Geometry: final body of the model. Coordinates: model frame, mm. A direction names the side the tool comes from. Give positions to 0.01 mm unless a question says otherwise; leave off trailing zeros. Write each loop counter-clockwise with the first axis right and the second up, starting at its lowest first coordinate (ties: lowest second). Pieces come first, ordered by that corner, then holes. Notation, with made-up numbers: (50, -18.75) -> (102, -18.75) arc R22 ccw to (102, 10.25) -> close; hole circle Ø1 at (3, -38.75). An arc over 180 degrees is marked (long way). Answer in a Markdown table with one row per item. Add a question column.
Item 1: Access query for faces 5 (the cylindrical face through (19.56, -1.13, -14.12)), 6 (the flat face through (-10.75, -1, -32)). Directions: +Z, -Z, +X, -X, +Y, -Y. A direction counts if a zero-diameter tool reaches every point of the face in a straight line with its end or side. Return the directions, or none.
Item 2: Section query C-C on x = -12.75. Output: boundary loops of the cut face in (y, z).
Item 3: Section query B-B on y = -1.7. State how many separate pieces and enclosed holes the cut face has, plus the area to 3 significant figures.
Item 4: First-contact query: P1, Ø4, axis at x = 12.75, z = 64, coming from the +Y side; P2, Ø0.7, axis at x = 2, y = -1, coming from the +Z side; P3, Ø1.1, axis at y = -1, z = 36, coming from the -X side; P4, Ø1.1, axis at x = -4, y = -1.5, coming from the -Z side. Flat tips, straight axial feed; report the tip coordinate or a pass-through.
Item 5: Draft query along X for faces 1 (the flat face through (6.095, -1.127, -41.717)), 2 (the cylindrical face through (-9.85, -1.13, -16.36)), 3 (the flat face through (-6.095, -1.127, 41.717)), 4 (the cylindrical face through (14.473, -1.127, 70.785)). Return one class per face: +X half, -X half, draft (parallel to the pull), parting line (faces both ways), or undercut.
Item 6: Material intervals for probe 1 along X at (y, z) = (-1.15, 12.5); probe 2 along Z at (x, y) = (-5, -1.65); probe 3 along Z at (x, y) = (6.5, -1.35), sorted ascending. Write a range as from..to.
Item 7: Section query A-A on z = 0. Output: boundary loops of the cut face in (x, y).
Item 8: Section query D-D on x = 0. Output: boundary loops of the cut face in (y, z), plus the area to 3 significant figures.
```python
from build123d import *

# Parameters (mm, degrees)
SKETCH1_R           = 2.1
SKETCH1_R_2         = 10
BOSS_EXTRUDE1_DEPTH = 2.286


with BuildPart() as part:
    # Sketch1 → Boss-Extrude1 (new body)
    with BuildSketch(Plane(origin=(0, 0, 0), x_dir=(1, 0, 0), z_dir=(0, 1, 0))):
        with BuildLine():
            Line((6.476876236, -67.106109825), (-19.023123764, -15.606109825))
            ThreePointArc((-19.023123764, -15.606109825), (-19.565858946, -14.095013112), (-19.75, -12.5))
            Line((-19.75, -12.5), (-19.75, 64))
            ThreePointArc((-19.75, 64), (-14.345013112, 70.815858946), (-6.476876236, 67.106109825))
            Line((-6.476876236, 67.106109825), (19.023123764, 15.606109825))
            ThreePointArc((19.023123764, 15.606109825), (19.565858946, 14.095013112), (19.75, 12.5))
            Line((19.75, 12.5), (19.75, -64))
            ThreePointArc((19.75, -64), (14.345013112, -70.815858946), (6.476876236, -67.106109825))
        make_face()
        with Locations(Location((-12.75, 64, 0), (0, 0, 270))):
            Circle(SKETCH1_R, mode=Mode.SUBTRACT)
        with Locations(Location((-12.75, 12.5, 0), (0, 0, 270))):
            Circle(SKETCH1_R, mode=Mode.SUBTRACT)
        with Locations(Location((12.75, 12.5, 0), (0, 0, 270))):
            Circle(SKETCH1_R, mode=Mode.SUBTRACT)
        with Locations(Location((12.75, -12.5, 0), (0, 0, 270))):
            Circle(SKETCH1_R, mode=Mode.SUBTRACT)
        with Locations(Location((12.75, -64, 0), (0, 0, 270))):
            Circle(SKETCH1_R, mode=Mode.SUBTRACT)
        with Locations(Location((-12.75, -12.5, 0), (0, 0, 270))):
            Circle(SKETCH1_R, mode=Mode.SUBTRACT)
        with Locations(Location((0, 0, 0), (0, 0, 270))):
            Circle(SKETCH1_R_2, mode=Mode.SUBTRACT)
        with BuildLine():
            Line((-5.061518387, 46.218659407), (8.004121842, 19.831189925))
            ThreePointArc((8.004121842, 19.831189925), (7.864519372, 16.917844789), (5.315640229, 15.5))
            Line((5.315640229, 15.5), (-7.75, 15.5))
            ThreePointArc((-7.75, 15.5), (-9.871320344, 16.378679656), (-10.75, 18.5))
            Line((-10.75, 18.5), (-10.75, 44.887469482))
            ThreePointArc((-10.75, 44.887469482), (-8.433577048, 47.808551887), (-5.061518387, 46.218659407))
        make_face(mode=Mode.SUBTRACT)
        with BuildLine():
            Line((5.061518387, -46.218659407), (-8.004121842, -19.831189925))
            ThreePointArc((-8.004121842, -19.831189925), (-7.864519372, -16.917844789), (-5.315640229, -15.5))
            Line((-5.315640229, -15.5), (7.75, -15.5))
            ThreePointArc((7.75, -15.5), (9.871320344, -16.378679656), (10.75, -18.5))
            Line((10.75, -18.5), (10.75, -44.887469482))
            ThreePointArc((10.75, -44.887469482), (8.433577048, -47.808551887), (5.061518387, -46.218659407))
        make_face(mode=Mode.SUBTRACT)
    extrude(amount=-BOSS_EXTRUDE1_DEPTH)


solid = part.part
```
Findings below:
| question | item | result |
|---|---|---|
| 1 | face 5 | -Z, +X, +Y, -Y |
| 1 | face 6 | +Y, -Y |
| 2 | outline | (-2.29, -71) -> (0, -71) -> (0, -66.1) -> (-2.29, -66.1) -> close; (-2.29, -61.9) -> (0, -61.9) -> (0, -14.6) -> (-2.29, -14.6) -> close; (-2.29, -10.4) -> (0, -10.4) -> (0, 10.4) -> (-2.29, 10.4) -> close; (-2.29, 14.6) -> (0, 14.6) -> (0, 28.28) -> (-2.29, 28.28) -> close |
| 3 | separate pieces | 1 |
| 3 | enclosed holes | 9 |
| 3 | area | 2,770 mm^2 |
| 4 | P1 | passes through |
| 4 | P2 | stops at z = 58.77 |
| 4 | P3 | stops at x = -9.2 |
| 4 | P4 | stops at z = -63.21 |
| 5 | face 1 | +X half |
| 5 | face 2 | undercut |
| 5 | face 3 | -X half |
| 5 | face 4 | parting line |
| 6 | probe 1 | x = -19.75..-14.85, -10.65..10.65, 14.85..19.75 |
| 6 | probe 2 | z = -64.12..-46.09, -15.5..-8.66, 8.66..15.5, 25.9..43.93 |
| 6 | probe 3 | z = -40.9..-22.87, -15.74..-7.6, 7.6..15.5, 47.61..67.15 |
| 7 | outline | (-19.75, -2.29) -> (-10, -2.29) -> (-10, 0) -> (-19.75, 0) -> close; (10, -2.29) -> (19.75, -2.29) -> (19.75, 0) -> (10, 0) -> close |
| 8 | outline | (-2.29, -54.03) -> (0, -54.03) -> (0, -36) -> (-2.29, -36) -> close; (-2.29, -15.5) -> (0, -15.5) -> (0, -10) -> (-2.29, -10) -> close; (-2.29, 10) -> (0, 10) -> (0, 15.5) -> (-2.29, 15.5) -> close; (-2.29, 36) -> (0, 36) -> (0, 54.03) -> (-2.29, 54.03) -> close |
| 8 | area | 108 mm^2 |
